Input: part model. Units: mm. Frame: model coordinates. Face numbers are marked on the shaded views. Round coordinates to 2 decimals unless told otherwise and drop trailing zeros. Order: outer loops, then holes, each group sorted by start corner. A loop starts at its lowest first (then second) coordinate and runs counter-clockwise, first axis right, second up.
Item 1: Cut plane A-A on z = 0. Output: boundary loops of the cut face in (x, y), then the cut area to 3 significant figures.
Item 2: Mould query, pull axis Z, two halves, no side actions, for the marked faces 1, 2 and 3. Classes: released by +Z, released by -Z, zero draft, split by the parting line, or undercut.
Item 3: Line query: L1, parallel to Y at x = 8.5, z = 0; L2, parallel to X at y = 15.5, z = -8; L3, parallel to Z at x = 6.75, y = 8.5. Output: solid intervals per line, ascending.
Item 4: First-contact query: pin 1 (8 mm diameter, centred on x = 1, z = 12, fed in from +Y); pin 2 (3 mm diameter, centred on x = 3.5, z = 13, fed in from -Y); pin 3 (4 mm diameter, centred on x = 10.5, y = -6, fed in from +Z). Flat tips, straight axial feed; report the tip coordinate or a pass-through.
Item 5: Cut plane C-C on x = 9. Output: boundary loops of the cut face in (y, z), then the cut area to 3 significant figures.
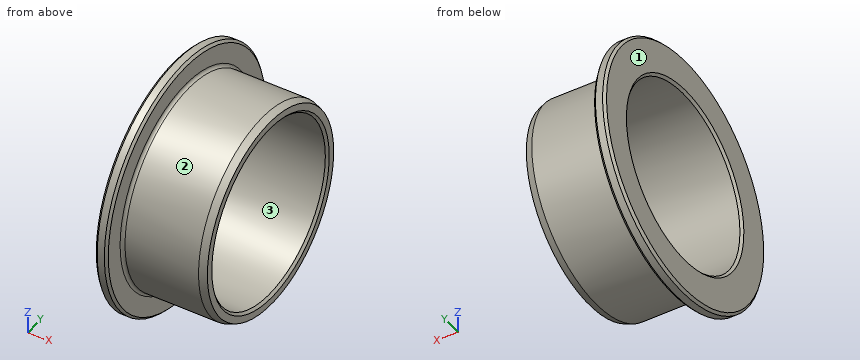
```python
from build123d import *

# Parameters (mm, degrees)
CONG_2_R         = 0.5
CHANFREIN1_SIZE  = 0.4
CHANFREIN3_SIZE  = 1.2
CHANFREIN3_SIZE2 = 0.436764281


with BuildPart() as part:
    # Esquisse1 → Base-Révolution (revolve)
    with BuildSketch(Plane.XY, mode=Mode.PRIVATE) as base_r_volution_sk:
        Polygon((-2, 15), (-2, 21), (0, 21), (0, 17), (14, 17), (14, 15), align=None)
    revolve(base_r_volution_sk.sketch.rotate(Axis((-5.312682662, 0, 0), (1, 0, 0)), 90), axis=Axis((-5.312682662, 0, 0), (1, 0, 0)))

    # Congé2
    cong_2_edges = [part.edges().sort_by_distance(p)[0] for p in [
        (0, 0, -17),
    ]]
    fillet(cong_2_edges, radius=CONG_2_R)

    # Chanfrein1
    chanfrein1_edges = [part.edges().sort_by_distance(p)[0] for p in [
        (0, 0, -21),
        (-2, 0, -21),
        (-2, 0, -15),
        (14, 0, -15),
    ]]
    chamfer(chanfrein1_edges, length=CHANFREIN1_SIZE)

    # Chanfrein3
    chanfrein3_edges = [part.edges().sort_by_distance(p)[0] for p in [
        (14, 0, -17),
    ]]
    chanfrein3_side = [part.faces().sort_by_distance(p)[0] for p in [
        (7.25, 0, -17),
    ]]
    chamfer(chanfrein3_edges, length=CHANFREIN3_SIZE, length2=CHANFREIN3_SIZE2, reference=chanfrein3_side[0])


solid = part.part
```
From the geometry:
1. outline: (-2, -20.6) - (-1.6, -21) - (-0.4, -21) - (0, -20.6) - (0, -17.5) arc R0.5 cw to (0.5, -17) - (12.8, -17) - (14, -16.56) - (14, -15.4) - (13.6, -15) - (-1.6, -15) - (-2, -15.4) - close; (-2, 15.4) - (-1.6, 15) - (13.6, 15) - (14, 15.4) - (14, 16.56) - (12.8, 17) - (0.5, 17) arc R0.5 cw to (0, 17.5) - (0, 20.6) - (-0.4, 21) - (-1.6, 21) - (-2, 20.6) - close
1. area: 78.9 mm2
2. face 1: zero draft
2. face 2: split by the parting line
2. face 3: undercut
3. L1: y = -17 to -15, 15 to 17
3. L2: x = -2 to 0
3. L3: z = -14.72 to -12.36, 12.36 to 14.72
4. pin 1: stops at y = 19.31
4. pin 2: stops at y = -12.52
4. pin 3: stops at z = 16.52
5. outline: circle Ø34 at (0, 0); hole circle Ø30 at (0, 0)
5. area: 201 mm2
